Autodesk Inventor part; units mm, degrees
ref_plane "YZ Plane" through (0, 0, 0) normal (1, 0, 0) x (0, 1, 0)
ref_plane "XZ Plane" through (0, 0, 0) normal (0, 1, 0) x (-1, 0, 0)
ref_plane "XY Plane" through (0, 0, 0) normal (0, 0, 1) x (1, 0, 0)
sketch "Sketch1" plane through (0, 0, 0) normal (0, 0, 1) x (1, 0, 0)
  line L0 (-40, 40) -> (40, 40)
  line L1 (40, 40) -> (40, -40)
  line L2 (40, -40) -> (-40, -40)
  line L3 (-40, -40) -> (-40, 40)
  line L4 (-40, 40) -> (40, -40) construction
  line L5 (40, 40) -> (-40, -40) construction
  point P0 (0, 0)
  dimension "d0" = 80
  dimension "d1" = 80
extrude "Extrusion1" add sketch "Sketch1" along normal blind 50
sketch "Sketch2" plane through (0, 0, 50) normal (0, 0, 1) x (1, 0, 0)
  circle A0 centre (0, 0) radius 25
  circle A1 centre (0, 0) radius 20
  dimension "d4" = 50
  dimension "d5" = 5
extrude "Extrusion2" add sketch "Sketch2" along normal blind 50
sketch "Sketch3" plane through (0, 0, 0) normal (0, 0, -1) x (-1, 0, 0)
  line L0 (-35, 35) -> (35, 35)
  line L1 (35, 35) -> (35, -35)
  line L2 (35, -35) -> (-35, -35)
  line L3 (-35, -35) -> (-35, 35)
  line L4 (-35, 35) -> (35, -35) construction
  line L5 (35, 35) -> (-35, -35) construction
  point P0 (0, 0)
  dimension "d8" = 70
  dimension "d9" = 70
sketch "Sketch4" plane through (0, 0, 0) normal (0, 0, -1) x (-1, 0, 0)
  line L0 (-40, 40) -> (40, 40)
  circle A0 centre (-35.0076, 34.9903) radius 3
  circle A1 centre (-34.4032, -35.1275) radius 3
  circle A2 centre (35.116, -34.8993) radius 3
  circle A3 centre (34.0977, 35.3717) radius 3
  point P0 (0, 0)
  dimension "d10" = 6
  dimension "d11" = 6
  dimension "d12" = 6
  dimension "d13" = 6
extrude "Extrusion3" cut sketch "Sketch4" against normal blind 50
fillet "Fillet1" radius 2 4 edges at (0, 40, 50) (40, 0, 50) (0, -40, 50) (-40, 0, 50)
thread "Thread1"
thread "Thread2"
thread "Thread3"
thread "Thread4"
thread "Thread5"
extrude "Extrusion4" add sketch "Sketch3" along normal blind 20 from surface at -50
sketch "Sketch5" plane through (0, 0, 50) normal (0, 0, 1) x (1, 0, 0)
  point P0 (0, 0)
Can you work these out from the model? Positions are in its coordinate system, mm. A direction names the side the tool comes from. Coordinates: 2 decimals unless noted, no trailing zeros. Write each loop counter-clockwise with the first axis right and the second up, starting at its lowest first coordinate (ties: lowest second). Pieces come first, ordered by that corner, then holes. Notation, with made-up numbers: (-22.75, 81) -> (29.25, 81) arc R31 ccw to (29.25, 107) -> close; hole circle Ø4 at (72, 45). An arc over 180 degrees is marked (long way). Write each question's results on one line, items separated by ' | '. Start each with the question number.
Q1. If I drill on probe 1 along Y at (x, z) = (-34.5, 21.5); probe 2 along Z at (x, y) = (-16, -31.5); probe 3 along Y at (x, z) = (-11.5, 81), over which ranges is the centre line in solid material (lowest first)?
Q2. Imagine slicing it at A-A (x = 0). Write out the boundary of the cut face in (y, z), then the cut area to 3 significant figures.
Q3. Imagine slicing it at C-C (z = 57). Write out the boundary of the cut face in (x, y), then the cut area to 3 significant figures.
Q4. I'm going to push flat-ended pins straight in: pin 1 (6 mm diameter, centred on x = -23.5, z = 84, fed in from -Y); pin 2 (12 mm diameter, centred on x = -25.5, z = 68.5, fed in from -Y); pin 3 (3.5 mm diameter, centred on x = 35.01, y = 34.99, fed in from -Z). Where does each tip first touch, or does it pass through?
Q5. We'd pull the mould along Y, two halves only. Please class faces 4 (the face through (40, 1, 24)), 5 (the face through (23.846, -7.509, 74.65)), 6 (the face through (1, -40, 24)), 7 (the face through (-34, -34, 30)): +Y half, -Y half, draft (parallel to the pull), parting line (faces both ways), or undercut.
Q6. On a 3-axis mill with a long thin cutter (end or side, diameter ignored), from which of +Z, -Z, +X, -X, +Y, -Y can I reach the whole of each face in a straight line? I mean faces 1 (the face through (0, 0, 50)), 2 (the face through (-34, -35, 40)), 3 (the face through (-33, 34, 30)). Say none if no direction works.
Q7. Imagine slicing it at D-D (x = -28.5). Write out the boundary of the cut face in (y, z), then the cut area to 3 significant figures.
Taken from the geometry:
1) probe 1: y = -40 to -37.84, -31.96 to 32.4, 38.34 to 40 | probe 2: z = 0 to 50 | probe 3: y = -22.2 to -16.36, 16.36 to 22.2
2) outline: (-40, 0) -> (40, 0) -> (40, 48) arc R2 ccw to (38, 50) -> (25, 50) -> (25, 100) -> (20, 100) -> (20, 50) -> (-20, 50) -> (-20, 100) -> (-25, 100) -> (-25, 50) -> (-38, 50) arc R2 ccw to (-40, 48) -> close | area: 4,500 mm^2
3) outline: circle Ø50 at (0, 0); hole circle Ø40 at (0, 0) | area: 707 mm^2
4) pin 1: stops at y = -14.31 | pin 2: stops at y = -15.64 | pin 3: stops at z = 30
5) face 4: draft | face 5: parting line | face 6: -Y half | face 7: undercut
6) face 1: +Z | face 2: +Z, -Z | face 3: -Z
7) outline: (-40, 0) -> (40, 0) -> (40, 48) arc R2 ccw to (38, 50) -> (-38, 50) arc R2 ccw to (-40, 48) -> close | area: 4,000 mm^2
